```python
from build123d import *

# Parameters (mm, degrees)
F0_R     = 8.5
F1_DEPTH = 10
F2_SIZE  = 1
F4_DEPTH = 25
F6_COUNT = 5
F7_R     = 30
F7_R_2   = 14
F8_DEPTH = 25


with BuildPart() as f1:
    # F0 (on Top) → F1 (new body)
    with BuildSketch(Plane.XY):
        Circle(F0_R)
    extrude(amount=F1_DEPTH)

    # F2
    f2_edges = [f1.edges().sort_by_distance(p)[0] for p in [
        (-8.5, 0, 10),
    ]]
    chamfer(f2_edges, length=F2_SIZE)

    # F3 (on Right) → F4 (join)
    with BuildSketch(Plane.YZ):
        with BuildLine():
            Line((5, 8.8), (5, 9))
            ThreePointArc((5, 9), (-1.7082039325, 6.4161984871), (-4.9498743711, 0))
            Line((-4.9498743711, 0), (-4.7488460856, 0))
            ThreePointArc((-4.7488460856, 0), (-1.5665820638, 6.2746133918), (5, 8.8))
        make_face()
    extrude(amount=F4_DEPTH)

    # F6: F1 ×5 about axis
    f6_axis = Axis((0, 0, 8.4288474172), (0, 0, 1))


with BuildPart() as f1_1:
    add(f1.part)
    for i in range(1, F6_COUNT):
        add(f1.part.rotate(f6_axis, i * 360 / F6_COUNT))

    # F7 (on Top) → F8 (cut)
    with BuildSketch(Plane.XY):
        Circle(F7_R)
        Circle(F7_R_2, mode=Mode.SUBTRACT)
    extrude(amount=F8_DEPTH, mode=Mode.SUBTRACT)


solid = f1_1.part
```
The listing builds one solid part. Answer for the finished solid, in the listing's coordinates (mm). A direction names the side the tool comes from. Give positions to 0.01 mm unless a question says otherwise; leave off trailing zeros. Order: outer loops, then holes, each group sorted by start corner. A loop starts at its lowest first (then second) coordinate and runs counter-clockwise, first axis right, second up. Notation, with made-up numbers: (-25.5, 84.5) -> (5.5, 84.5) arc R14 ccw to (5.5, 104.5) -> close; hole circle Ø8 at (33, 64). An arc over 180 degrees is marked (long way). One line per item, written item: value.
1) Find section C-C, the plane z = 0.5. Determine the outline of the cut face in (x, y), plus the area to 3 significant figures.
Reported:
outline: (-13.49, -3.76) arc R14 ccw to (-13.43, -3.96) -> (-8.49, -0.38) arc R8.5 ccw to (-2.5, -8.12) -> (-0.59, -13.99) arc R14 ccw to (-0.38, -13.99) -> (-2.26, -8.19) arc R8.5 ccw to (6.95, -4.89) -> (13.12, -4.89) arc R14 ccw to (13.19, -4.68) -> (7.09, -4.68) arc R8.5 ccw to (6.8, 5.1) -> (8.7, 10.97) arc R14 ccw to (8.53, 11.1) -> (6.65, 5.3) arc R8.5 ccw to (-2.75, 8.04) -> (-7.74, 11.66) arc R14 ccw to (-7.92, 11.54) -> (-2.98, 7.96) arc R8.5 ccw to (-8.5, -0.13) -> close
area: 233 mm^2
2) Find the intervals of material crossed by line 1 (X direction, y = 4, z = 5.75); line 2 (X direction, y = -2.75, z = 4.25); line 3 (Y direction, x = 12.25, z = 1.25), in increasing order.
Reported:
line 1: x = -7.5 to 7.5
line 2: x = -9.76 to -9.36, -8.04 to 8.04
line 3: y = -4.74 to -4.54
3) Find section B-B, the plane x = 12.25. Determine the outline of the cut face in (y, z).
Reported:
outline: (-4.95, 0) -> (-4.75, 0) arc R9.8 cw to (5, 8.8) -> (5, 9) arc R10 ccw to start
4) A tool of negligible diameter and unlimited length cuts with its end or side. For faces 4 (the cylindrical face through (-9.369, -4.778, 6.207)), 5 (the cylindrical face through (-7.445, 7.426, 6.485)), 6 (the cylindrical face through (1.658, -10.384, 6.485)), from which of +Z, -Z, +X, -X, +Y, -Y can it reach the whole face along a straight path? Write none if from no direction.
Reported:
face 4: -Z, -Y
face 5: +Z, +Y
face 6: +Z, -Y
5) Determine the mould class of faces 1 (the cylindrical face through (-7.44, 7.43, 6.21)), 2 (the flat face through (0, 0, 0)), 3 (the cylindrical face through (-0.335, 8.493, 4.437)) for opening direction X: pulls with the +X half, pulls with the -X half, needs draft (parallel to the pull), parting line crosses it, or undercut.
Reported:
face 1: pulls with the -X half
face 2: needs draft
face 3: undercut
6) Flat-ended cylindrical pins translate along their axes: P1, Ø3, axis at x = 1.5, z = 7.5, coming from the +Y side; P2, Ø4, axis at y = 0.5, z = 2, coming from the -X side; P3, Ø3, axis at y = 4, z = 7.5, coming from the +X side. Find the tip coordinate at first contact, or state that the pin passes through.
Reported:
P1: stops at y = 13.99
P2: stops at x = -9.95
P3: stops at x = 13.68
7) Find section A-A, the plane z = 4.75. Determine the outline of the cut face in (x, y), plus the area to 3 significant figures.
Reported:
outline: (-12.9, -5.44) arc R14 ccw to (-12.8, -5.67) -> (-8.18, -2.31) arc R8.5 ccw to (-0.59, -8.48) -> (1.19, -13.95) arc R14 ccw to (1.44, -13.93) -> (-0.33, -8.49) arc R8.5 ccw to (7.88, -3.18) -> (13.63, -3.18) arc R14 ccw to (13.69, -2.94) -> (7.98, -2.94) arc R8.5 ccw to (5.46, 6.51) -> (7.24, 11.98) arc R14 ccw to (7.02, 12.11) -> (5.26, 6.68) arc R8.5 ccw to (-4.51, 7.21) -> (-9.16, 10.59) arc R14 ccw to (-9.35, 10.42) -> (-4.73, 7.06) arc R8.5 ccw to (-8.25, -2.06) -> close
area: 234 mm^2
